Model file for the job. Use its own axes, mm. Give positions to 0.01 mm unless a question says otherwise; leave off trailing zeros. Write each loop counter-clockwise with the first axis right and the second up, starting at its lowest first coordinate (ties: lowest second). Pieces come first, ordered by that corner, then holes.
Solid Edge part; units mm, degrees
sketch "Sketch1" plane through (0, 0, 0) normal (0, 0, 1) x (1, 0, 0)
  line L0 (46.5, -60) -> (46.5, 60)
  line L1 (46.5, 60) -> (-46.5, 60)
  line L2 (-46.5, 60) -> (-46.5, -60)
  line L3 (-46.5, -60) -> (46.5, -60)
extrude "Protrusion1" add sketch "Sketch1" along normal blind 2
sketch "Sketch2" plane through (0, 0, 2) normal (0, 0, 1) x (1, 0, 0)
  circle A0 centre (-34, 25.5) radius 3.5
  line L0 (-28.5, 5.5) -> (-39.5, 5.5)
  line L1 (-39.5, 5.5) -> (-39.5, -5.5)
  line L2 (-39.5, -5.5) -> (-28.5, -5.5)
  line L3 (-28.5, -5.5) -> (-28.5, 5.5)
  circle A1 centre (-17, 25.5) radius 3.5
  line L4 (-11.5, 5.5) -> (-22.5, 5.5)
  line L5 (-22.5, 5.5) -> (-22.5, -5.5)
  line L6 (-22.5, -5.5) -> (-11.5, -5.5)
  line L7 (-11.5, -5.5) -> (-11.5, 5.5)
  circle A2 centre (0, 25.5) radius 3.5
  line L8 (5.5, 5.5) -> (-5.5, 5.5)
  line L9 (-5.5, 5.5) -> (-5.5, -5.5)
  line L10 (-5.5, -5.5) -> (5.5, -5.5)
  line L11 (5.5, -5.5) -> (5.5, 5.5)
  circle A3 centre (17, 25.5) radius 3.5
  line L12 (22.5, 5.5) -> (11.5, 5.5)
  line L13 (11.5, 5.5) -> (11.5, -5.5)
  line L14 (11.5, -5.5) -> (22.5, -5.5)
  line L15 (22.5, -5.5) -> (22.5, 5.5)
  circle A4 centre (34, 25.5) radius 3.5
  line L16 (39.5, 5.5) -> (28.5, 5.5)
  line L17 (28.5, 5.5) -> (28.5, -5.5)
  line L18 (28.5, -5.5) -> (39.5, -5.5)
  line L19 (39.5, -5.5) -> (39.5, 5.5)
extrude "Cutout1" cut sketch "Sketch2" against normal up to next
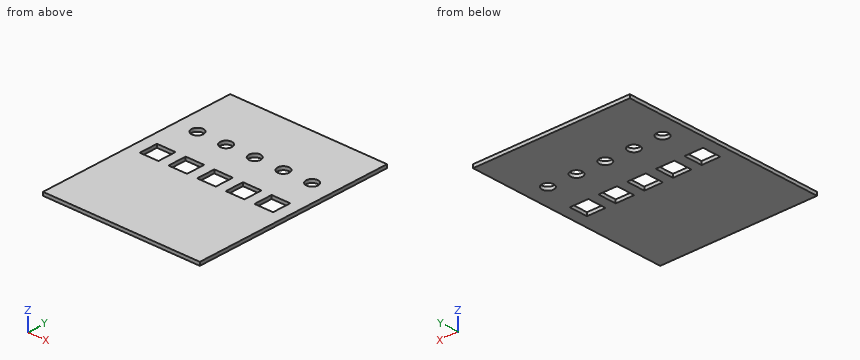
1. Slice it at D-D, the plane y = 25.5. Write the cut outline in (x, z).
Calculated:
outline: (-46.5, 0) - (-37.5, 0) - (-37.5, 2) - (-46.5, 2) - close; (-30.5, 0) - (-20.5, 0) - (-20.5, 2) - (-30.5, 2) - close; (-13.5, 0) - (-3.5, 0) - (-3.5, 2) - (-13.5, 2) - close; (3.5, 0) - (13.5, 0) - (13.5, 2) - (3.5, 2) - close; (20.5, 0) - (30.5, 0) - (30.5, 2) - (20.5, 2) - close; (37.5, 0) - (46.5, 0) - (46.5, 2) - (37.5, 2) - close
2. Slice it at A-A, the plane y = -3.5. Write the cut outline in (x, z).
Calculated:
outline: (-46.5, 0) - (-39.5, 0) - (-39.5, 2) - (-46.5, 2) - close; (-28.5, 0) - (-22.5, 0) - (-22.5, 2) - (-28.5, 2) - close; (-11.5, 0) - (-5.5, 0) - (-5.5, 2) - (-11.5, 2) - close; (5.5, 0) - (11.5, 0) - (11.5, 2) - (5.5, 2) - close; (22.5, 0) - (28.5, 0) - (28.5, 2) - (22.5, 2) - close; (39.5, 0) - (46.5, 0) - (46.5, 2) - (39.5, 2) - close
3. Slice it at B-B, the plane z = 1.6. State how many separate pieces and enclosed holes the cut face has, and give its area (3 significant figures).
Calculated:
separate pieces: 1
enclosed holes: 10
area: 10,400 mm2
4. Pin check, flat tip, straight feed: P1, Ø6.5, axis at x = -34, y = 25.5, coming from the -Z side. Stop position of the tip, or through.
Calculated:
P1: passes through
5. Slice it at C-C, the plane x = -17. Write the cut outline in (y, z), and give its area (3 significant figures).
Calculated:
outline: (-60, 0) - (-5.5, 0) - (-5.5, 2) - (-60, 2) - close; (5.5, 0) - (22, 0) - (22, 2) - (5.5, 2) - close; (29, 0) - (60, 0) - (60, 2) - (29, 2) - close
area: 204 mm2
6. Probe probe 1 along Y at (x, z) = (34, 1.05); probe 2 along X at (y, z) = (-3, 0.9); probe 3 along Y at (x, z) = (-2.5, 0.45). List the from-to ranges inside material, lowest first.
Calculated:
probe 1: y = -60 to -5.5, 5.5 to 22, 29 to 60
probe 2: x = -46.5 to -39.5, -28.5 to -22.5, -11.5 to -5.5, 5.5 to 11.5, 22.5 to 28.5, 39.5 to 46.5
probe 3: y = -60 to -5.5, 5.5 to 23.05, 27.95 to 60
